Autodesk Inventor part; units mm, degrees
ref_plane "YZ Plane" through (0, 0, 0) normal (1, 0, 0) x (0, 1, 0)
ref_plane "XZ Plane" through (0, 0, 0) normal (0, 1, 0) x (-1, 0, 0)
ref_plane "XY Plane" through (0, 0, 0) normal (0, 0, 1) x (1, 0, 0)
sketch "Sketch_1" plane through (0, 0, 0) normal (1, 0, 0) x (0, 1, 0)
  line L0 (1, 57) -> (0, 56)
  line L1 (0, 56) -> (0, 1)
  arc A0 (0, 1) -> (1, 0) centre (1, 1) ccw
  line L2 (1, 0) -> (56, 0)
  line L3 (56, 0) -> (57, 1)
  line L4 (57, 1) -> (57, 5)
  line L5 (57, 5) -> (5, 57)
  line L6 (5, 57) -> (1, 57)
extrude "Extrusion1" add sketch "Sketch_1" along normal mid plane 28
sketch "Sketch_2" plane through (-9, 0, 0) normal (1, 0, 0) x (0, 0, -1)
  line L0 (-56, 6) -> (-7, 6)
  arc A0 (-7, 6) -> (-6, 7) centre (-7, 7) ccw
  line L1 (-6, 7) -> (-6, 56)
  line L2 (-6, 56) -> (-56, 6)
extrude "Extrusion2" cut sketch "Sketch_2" along normal blind 23
sketch "Sketch_3" plane through (0, 0, 0) normal (1, 0, 0) x (0, 1, 0)
  line L0 (0, 4.6669) -> (0, 1)
  arc A0 (0, 1) -> (1, 0) centre (1, 1) ccw
  line L1 (1, 0) -> (4.6669, 0)
  line L2 (4.6669, 0) -> (2.687, 1.9799)
  line L3 (2.687, 1.9799) -> (1.9799, 1.2728)
  line L4 (1.9799, 1.2728) -> (1.2728, 1.9799)
  line L5 (1.2728, 1.9799) -> (1.9799, 2.687)
  line L6 (1.9799, 2.687) -> (0, 4.6669)
extrude "Extrusion3" cut sketch "Sketch_3" along normal mid plane 12
sketch "Sketch_4" plane through (0, 0, 0) normal (1, 0, 0) x (0, 1, 0)
  line L0 (53.8787, 2.1213) -> (51.7574, 0)
  line L1 (51.7574, 0) -> (56, 0)
  line L2 (56, 0) -> (53.8787, 2.1213)
extrude "Extrusion4" cut sketch "Sketch_4" along normal mid plane 12
sketch "Sketch_5" plane through (0, 0, 0) normal (1, 0, 0) x (0, 1, 0)
  line L0 (0, 56) -> (0, 51.7574)
  line L1 (0, 51.7574) -> (2.1213, 53.8787)
  line L2 (2.1213, 53.8787) -> (0, 56)
extrude "Extrusion5" cut sketch "Sketch_5" along normal mid plane 12
sketch "Sketch_6" plane through (0, 0, 0) normal (1, 0, 0) x (0, 1, 0)
  line L0 (55.2929, 0.7071) -> (53.313, -1.2728)
  line L1 (53.313, -1.2728) -> (54.0201, -1.9799)
  line L2 (54.0201, -1.9799) -> (56, 0)
  line L3 (56, 0) -> (55.2929, 0.7071)
extrude "Extrusion6" add sketch "Sketch_6" along normal mid plane 8
sketch "Sketch22" plane through (0, -2.1213, 2.1213) normal (0, -0.7071, 0.7071) x (1, 0, 0)
  line L0 (-4, 3.3) -> (-4, 0.2)
  line L1 (-4, 0.2) -> (4, 0.2)
  line L2 (4, 0.2) -> (4, 3.3)
  line L3 (4, 3.3) -> (-4, 3.3)
extrude "Extrusion7" add sketch "Sketch22" against normal blind 1
sketch "Sketch25" plane through (0, 2.1213, -2.1213) normal (0, 0.7071, -0.7071) x (-1, 0, 0)
  line L0 (-4, 3.3) -> (-4, 0.2)
  line L1 (-4, 0.2) -> (4, 0.2)
  line L2 (4, 0.2) -> (4, 3.3)
  line L3 (4, 3.3) -> (-4, 3.3)
extrude "Extrusion8" add sketch "Sketch25" against normal blind 1
sketch "Sketch_7" plane through (0, 0, 0) normal (1, 0, 0) x (0, 1, 0)
  line L0 (0, 56) -> (-1.9799, 54.0201)
  line L1 (-1.9799, 54.0201) -> (-1.2728, 53.313)
  line L2 (-1.2728, 53.313) -> (0.7071, 55.2929)
  line L3 (0.7071, 55.2929) -> (0, 56)
extrude "Extrusion9" add sketch "Sketch_7" along normal mid plane 8
sketch "Sketch_8" plane through (-9, 0, 0) normal (1, 0, 0) x (0, 0, -1)
  line L0 (-57, 3.7759) -> (-57, 1)
  line L1 (-57, 1) -> (-56, 0)
  line L2 (-56, 0) -> (-52.5, 0)
  line L3 (-52.5, 0) -> (-57, 3.7759)
extrude "Extrusion10" cut sketch "Sketch_8" along normal mid plane 4
sketch "Sketch_9" plane through (-9, 0, 0) normal (1, 0, 0) x (0, 0, -1)
  line L0 (-3.7759, 57) -> (0, 52.5)
  line L1 (0, 52.5) -> (0, 56)
  line L2 (0, 56) -> (-1, 57)
  line L3 (-1, 57) -> (-3.7759, 57)
extrude "Extrusion11" cut sketch "Sketch_9" along normal mid plane 4
sketch "Sketch_16" plane through (9, 0, 0) normal (1, 0, 0) x (0, 0, -1)
  line L0 (-13.0711, 6) -> (-7, 6)
  arc A0 (-7, 6) -> (-6, 7) centre (-7, 7) ccw
  line L1 (-6, 7) -> (-6, 13.0711)
  line L2 (-6, 13.0711) -> (-13.0711, 6)
extrude "Extrusion12" add sketch "Sketch_16" along normal mid plane 4
sketch "Sketch_10" plane through (9, 0, 0) normal (1, 0, 0) x (0, 0, -1)
  line L0 (-3.7759, 57) -> (0, 52.5)
  line L1 (0, 52.5) -> (0, 56)
  line L2 (0, 56) -> (-1, 57)
  line L3 (-1, 57) -> (-3.7759, 57)
extrude "Extrusion13" cut sketch "Sketch_10" along normal mid plane 4
sketch "Sketch_11" plane through (9, 0, 0) normal (1, 0, 0) x (0, 0, -1)
  line L0 (-57, 1) -> (-56, 0)
  line L1 (-56, 0) -> (-52.5, 0)
  line L2 (-52.5, 0) -> (-57, 3.7759)
  line L3 (-57, 3.7759) -> (-57, 1)
extrude "Extrusion14" cut sketch "Sketch_11" along normal mid plane 4
sketch "Sketch_12" plane through (0, 0, 0) normal (1, 0, 0) x (0, 1, 0)
  line L0 (21, 6) -> (10.2426, 6)
  line L1 (10.2426, 6) -> (4.4548, 0.2121)
  line L2 (4.4548, 0.2121) -> (4.6669, 0)
  line L3 (4.6669, 0) -> (21, 0)
  line L4 (21, 0) -> (21, 6)
extrude "Extrusion15" cut sketch "Sketch_12" along normal mid plane 6.2
sketch "Sketch_13" plane through (0, 0, 0) normal (1, 0, 0) x (0, 1, 0)
  line L0 (0, 21) -> (0, 4.6669)
  line L1 (0, 4.6669) -> (0.2121, 4.4548)
  line L2 (0.2121, 4.4548) -> (6, 10.2426)
  line L3 (6, 10.2426) -> (6, 21)
  line L4 (6, 21) -> (0, 21)
extrude "Extrusion16" cut sketch "Sketch_13" along normal mid plane 6.2
sketch "Sketch_14" plane through (0, 0, 0) normal (1, 0, 0) x (0, 1, 0)
  line L0 (40, 6) -> (34, 0)
  line L1 (34, 0) -> (51, 0)
  line L2 (51, 0) -> (51, 6)
  line L3 (51, 6) -> (40, 6)
extrude "Extrusion17" cut sketch "Sketch_14" along normal mid plane 6.2
sketch "Sketch_15" plane through (0, 0, 0) normal (1, 0, 0) x (0, 1, 0)
  line L0 (0, 51) -> (0, 34)
  line L1 (0, 34) -> (6, 40)
  line L2 (6, 40) -> (6, 51)
  line L3 (6, 51) -> (0, 51)
extrude "Extrusion18" cut sketch "Sketch_15" along normal mid plane 6.2
properties part number "14070_m"
CAD build for the part. Positions are in the model's coordinates, mm. A direction names the side the tool comes from. Give positions to 0.01 mm unless a question says otherwise; leave off trailing zeros. Order: outer loops, then holes, each group sorted by start corner. A loop starts at its lowest first (then second) coordinate and runs counter-clockwise, first axis right, second up. Notation, with made-up numbers: M 43.5,26.25 L 63.5,26.25 A19 cw 63.5,53.25 Z; hole C -21.75,31 d2. An arc over 180 degrees is marked long. Put each result on its own line as item: value. Start each with the question number.
(1) Drill centre lines: line 1 along X through (y, z) = (3, 16); line 2 along Z through (x, y) = (-0.75, 1); line 3 along X through (y, z) = (13.5, 41.5). Where is each one in solid material? Low to high.
(2) Saw through at B-B, the plane x = 12. Write the cut outline in (y, z).
(3) Which spindle directions (+Z, -Z, +X, -X, +Y, -Y) get a long thin tool onto all of the face, cutting with end or side? Do faces 1 (the flat face through (-11, 1, 55)), 2 (the flat face through (3.1, 44, 3)), 3 (the flat face through (-0.056, -0.297, 54.289)). Say none if no direction does.
(4) Saw through at D-D, the plane y = 28. Write the cut outline in (x, z), then the cut area to 3 significant figures.
(5) Saw through at A-A, the plane z = 47.5. Write the cut outline in (x, y).
(6) Saw through at C-C, the plane z = 35. Write the cut outline in (x, y).
(7) Mould opens along Y. For faces 4 (the flat face through (-0.084, 1.224, 3.443)), 5 (the flat face through (4, -1, 3)), 6 (the flat face through (-9.028, 1.862, 54.718)) say: +Y half, -Y half, draft (parallel to the pull), parting line (faces both ways), or undercut.
(8) Flat gauge pins, fed straight in: pin 1 Ø1 at (x, y) = (-5, 29.5) entering from +Z; pin 2 Ø1.5 at (y, z) = (43, 21.5) entering from +X; pin 3 Ø0.8 at (y, z) = (54.5, -1.5) entering from +X; pin 4 Ø3 at (x, y) = (0.5, 3) entering from -Z. Where does each tip first touch, or does it go through?
Check result:
1. line 1: x = -14 to -3.1, 3.1 to 14
1. line 2: z = 3.67 to 5.24, 21 to 35, 51 to 52.76, 55 to 57
1. line 3: x = -14 to -9
2. outline: M 0,1 A1 ccw 1,0 L 56,0 L 57,1 L 57,5 L 56,6 L 7,6 A1 cw 6,7 L 6,56 L 5,57 L 1,57 L 0,56 Z
3. face 1: +Z, -Y
3. face 2: -Z
3. face 3: none
4. outline: M -14,0 L 14,0 L 14,6 L -9,6 L -9,34 L -14,34 Z
4. area: 308 mm2
5. outline: M -14,0 L -3.1,0 L -3.1,6 L -9,6 L -9,14.5 L -14,14.5 Z; M 3.1,0 L 14,0 L 14,6 L 3.1,6 Z
6. outline: M -14,0 L -3.1,0 L -3.1,1 L 3.1,1 L 3.1,0 L 14,0 L 14,6 L -9,6 L -9,27 L -14,27 Z
7. face 4: undercut
7. face 5: draft
7. face 6: -Y half
8. pin 1: stops at z = 6
8. pin 2: passes through
8. pin 3: stops at x = 4
8. pin 4: stops at z = -1.98
